Autodesk Fusion 360 part; units mm, degrees
sketch "スケッチ1" plane through (0, 0, 0) normal (0, 0, 1) x (1, 0, 0)
  line L0 (-16.5, 22) -> (16.5, 22)
  line L1 (16.5, 22) -> (16.5, 0)
  line L2 (16.5, 0) -> (-16.5, 0)
  line L3 (-16.5, 0) -> (-16.5, 22)
  dimension "d7" = 22
  dimension "d8" = 33
extrude "押し出し1" add sketch "スケッチ1" along normal blind 2
sketch "スケッチ3" plane through (0, 0, 0) normal (0, 0, -1) x (1, 0, 0)
  line L0 (16.5, 0) -> (-16.5, 0)
  line L1 (-16.5, 0) -> (-16.5, -22)
  line L2 (-16.5, -22) -> (16.5, -22)
  line L3 (16.5, -22) -> (16.5, 0)
  arc A0 (-4.95, -13) -> (4.95, -13) centre (0, -13) ccw
  line L4 (16.5, -13) -> (-16.5, -13)
  dimension "d9" = 9.9
  dimension "d10" = 9
extrude "押し出し2" add sketch "スケッチ3" along normal blind 2 contours L1 L2 L3 A0 L4
sketch "スケッチ4" plane through (0, 0, -2) normal (0, 0, -1) x (1, 0, 0)
  line L0 (-4.95, -13) -> (-16.5, -13)
  line L1 (-16.5, -13) -> (-16.5, -22)
  line L2 (-16.5, -22) -> (16.5, -22)
  line L3 (16.5, -22) -> (16.5, -13)
  line L4 (16.5, -13) -> (4.95, -13)
  arc A0 (-4.95, -13) -> (4.95, -13) centre (0, -13) ccw
  line L5 (16.5, -22) -> (0.6, -22)
  line L6 (0.6, -22) -> (0.6, -13)
  line L7 (0.6, -13) -> (16.5, -13)
  line L8 (16.5, -13) -> (16.5, -22)
  line L9 (-16.5, -22) -> (-0.6, -22)
  line L10 (-0.6, -22) -> (-0.6, -13)
  line L11 (-0.6, -13) -> (-16.5, -13)
  line L12 (-16.5, -13) -> (-16.5, -22)
  dimension "d13" = 1.2
extrude "押し出し3" add sketch "スケッチ4" along normal blind 2
sketch "スケッチ5" plane through (0, 0, 0) normal (0, 0, -1) x (1, 0, 0)
  line L0 (4.95, -13) -> (16.5, -13)
  line L1 (16.5, -13) -> (16.5, 0)
  line L2 (16.5, 0) -> (-16.5, 0)
  line L3 (-16.5, 0) -> (-16.5, -13)
  line L4 (-16.5, -13) -> (-4.95, -13)
  arc A0 (-4.95, -13) -> (4.95, -13) centre (0, -13) ccw
  line L5 (-3.75, 0) -> (3.75, 0)
  line L6 (3.75, 0) -> (3.75, -18)
  line L7 (3.75, -18) -> (-3.75, -18)
  line L8 (-3.75, -18) -> (-3.75, 0)
  line L9 (0, -1.75) -> (0, -22.5)
  line L10 (3.75, -7) -> (16.5, -7)
  line L11 (-3.75, -7) -> (-16.5, -7)
  dimension "d17" = 7.5
  dimension "d18" = 11
  dimension "d19" = 11
sketch "スケッチ9" plane through (0, 13, 0) normal (0, -1, 0) x (1, 0, 0)
  line L0 (-4.95, 0) -> (-16.5, 0)
  line L1 (-16.5, 0) -> (-16.5, -4)
  line L2 (-16.5, -4) -> (-0.6, -4)
  line L3 (-0.6, -4) -> (-0.6, -2)
  line L4 (-0.6, -2) -> (-4.95, -2)
  line L5 (-4.95, -2) -> (-4.95, 0)
  line L6 (-2, -2) -> (2, -2)
  line L7 (2, -2) -> (2, -4)
  line L8 (2, -4) -> (-2, -4)
  line L9 (-2, -4) -> (-2, -2)
  line L10 (16.5, -4) -> (0.6, -4)
  dimension "d37" = 4
  dimension "d38" = 2
extrude "押し出し7" cut sketch "スケッチ9" against normal blind 1.5 contours L2 L3 L4 L6 L8 L9 | L3 L6 L7 L8 L10
sketch "スケッチ11" plane through (0, 22, 0) normal (0, 1, 0) x (-1, 0, 0)
  line L0 (16.5, -4) -> (16.5, 2)
  line L1 (16.5, 2) -> (-16.5, 2)
  line L2 (-16.5, 2) -> (-16.5, -4)
  line L3 (-16.5, -4) -> (16.5, -4)
  line L4 (16.5, 2) -> (-13.5, 2)
  line L5 (-13.5, 2) -> (-13.5, 12)
  line L6 (-13.5, 12) -> (16.5, 12)
  line L7 (16.5, 12) -> (16.5, 2)
  dimension "d49" = 10
ref_plane "作業平面1" through (0, 11, -1) normal (0, 1, 0) x (-1, 0, 0)
sketch "スケッチ13" plane through (0, 11, -1) normal (0, 1, 0) x (1, 0, 0)
  line L0 (16.5, -10) -> (-16.5, -10)
  line L1 (-16.5, -10) -> (-16.5, -3)
  line L2 (-16.5, -3) -> (16.5, -3)
  line L3 (16.5, -3) -> (16.5, -10)
  line L4 (16.5, 3) -> (16.5, -3)
  line L5 (-16.5, 3) -> (-16.5, -3)
  circle A0 centre (0, -6.5) radius 2.25
  dimension "d53" = 7
  dimension "d54" = 4.5
  dimension "d58" = 3.5
extrude "押し出し11" add sketch "スケッチ13" along normal blind -2 and the other way blind -8
sketch "Sketch17" plane through (16.5, 0, 0) normal (1, 0, 0) x (0, 1, 0)
  line L0 (22, -4) -> (22, 2)
  line L1 (22, 2) -> (19, 2)
  line L2 (19, 2) -> (19, 9)
  line L3 (19, 9) -> (9, 9)
  line L4 (9, 9) -> (9, 2)
  line L5 (9, 2) -> (0, 2)
  line L6 (0, 2) -> (0, 0)
  line L7 (0, 0) -> (13, 0)
  line L8 (13, 0) -> (13, -4)
  line L9 (13, -4) -> (22, -4)
  line L10 (11, 9) -> (17, 9)
  line L11 (17, 9) -> (17, 2)
  line L12 (17, 2) -> (11, 2)
  line L13 (11, 2) -> (11, 9)
extrude "Extrude15" cut sketch "Sketch17" against normal blind 400 contours L3 L10 L11 L12 L13
sketch "Sketch18" plane through (-16.5, 0, 0) normal (-1, 0, 0) x (0, -1, 0)
  line L0 (-11, 9) -> (-11, 2)
  line L1 (-11, 2) -> (-17, 2)
  line L2 (-17, 2) -> (-17, 9)
  line L3 (-17, 9) -> (-19, 9)
  line L4 (-19, 9) -> (-19, 2)
  line L5 (-19, 2) -> (-22, 2)
  line L6 (-22, 2) -> (-22, -4)
  line L7 (-22, -4) -> (-13, -4)
  line L8 (-13, -4) -> (-13, 0)
  line L9 (-13, 0) -> (0, 0)
  line L10 (0, 0) -> (0, 2)
  line L11 (0, 2) -> (-9, 2)
  line L12 (-9, 2) -> (-9, 9)
  line L13 (-9, 9) -> (-11, 9)
  line L14 (-9, 2) -> (0, 2)
  line L15 (0, 2) -> (0, 0)
  line L16 (0, 0) -> (-9, 0)
  line L17 (-9, 0) -> (-9, 2)
extrude "Extrude16" cut sketch "Sketch18" against normal blind 34 contours L9 L10 L11 L14 L15 L16 L17
sketch "Sketch19" plane through (0, 13, 0) normal (0, -1, 0) x (1, 0, 0)
  line L0 (2, -2) -> (2, -4)
  line L1 (2, -4) -> (16.5, -4)
  line L2 (16.5, -4) -> (16.5, 0)
  line L3 (16.5, 0) -> (4.95, 0)
  line L4 (4.95, 0) -> (4.95, -2)
  line L5 (4.95, -2) -> (2, -2)
  line L6 (0.6, -2) -> (16.5, -2)
  line L7 (-0.6, -2) -> (-16.5, -2)
  point P0 (12, -2)
  point P1 (-12, -2)
hole "Hole1" at (-12, 13, -2) at (12, 13, -2) direction (0, 1, 0) diameter 2.75 depth 5 tip angle 118
sketch "Sketch20" plane through (0, 9, 0) normal (0, -1, 0) x (1, 0, 0)
  circle A0 centre (0, 5.5) radius 2.25
  line L0 (16.5, 0) -> (16.5, 9)
  line L1 (16.5, 9) -> (-16.5, 9)
  line L2 (-16.5, 9) -> (-16.5, 0)
  line L3 (-16.5, 0) -> (16.5, 0)
  circle A1 centre (0, 5) radius 4
  curve L4
  curve L5
  curve L6
  curve L7
  line L8 (-16.5, 2.0263) -> (16.5, 2.0263)
  line L9 (16.5, 2.0263) -> (16.5, 0)
  line L10 (16.5, 0) -> (-16.5, 0)
  line L11 (-16.5, 0) -> (-16.5, 2.0263)
  line L12 (-4, 5) -> (-4, 2.0263)
  line L13 (4, 5) -> (4, 2.0263)
  point P0 (-16.5, 2)
extrude "Extrude17" cut sketch "Sketch20" against normal blind 150 contours L0 L1 A1 L8 L13 | L1 L2 A1 L8 L12
sketch "Sketch21" plane through (0, 0, -4) normal (0, 0, -1) x (1, 0, 0)
  line L0 (2, -13) -> (2, -14.5)
  line L1 (2, -14.5) -> (0.6, -14.5)
  line L2 (0.6, -14.5) -> (0.6, -17.9135)
  arc A0 (-0.6, -17.9135) -> (0.6, -17.9135) centre (0, -13) ccw
  line L3 (-0.6, -17.9135) -> (-0.6, -14.5)
  line L4 (-0.6, -14.5) -> (-2, -14.5)
  line L5 (-2, -14.5) -> (-2, -13)
  line L6 (-2, -13) -> (-16.5, -13)
  line L7 (-16.5, -13) -> (-16.5, -22)
  line L8 (-16.5, -22) -> (16.5, -22)
  line L9 (16.5, -22) -> (16.5, -13)
  line L10 (16.5, -13) -> (2, -13)
sketch "Sketch22" plane through (0, 0, 0) normal (0, 0, -1) x (1, 0, 0)
  line L0 (16.5, -9) -> (-16.5, -9)
  line L1 (-16.5, -9) -> (-16.5, -13)
  line L2 (-16.5, -13) -> (-4.95, -13)
  arc A0 (-4.95, -13) -> (4.95, -13) centre (0, -13) ccw
  line L3 (4.95, -13) -> (16.5, -13)
  line L4 (16.5, -13) -> (16.5, -9)
  circle A1 centre (0, -13) radius 9
extrude "Extrude18" cut sketch "Sketch22" against normal blind 10 contours L0 L3 L4 A1 | L0 L1 L2 A1
move_face "OffsetFaces1" offset -1 1 faces at (16.5, 17.3333, -2)
move_face "OffsetFaces2" offset -0.5 1 faces at (15.5, 17.3333, -2)
move_face "OffsetFaces3" offset -1.5 1 faces at (-16.5, 17.3333, -2)
move_face "OffsetFaces4" offset 1 1 faces at (5, 22, 0)
move_face "OffsetFaces5" offset -1 1 faces at (5, 23, 0)
Here's how the part is built. I have some questions about the finished solid (model axes, mm). A direction names the side the tool comes from. Coordinates: 2 decimals unless noted, no trailing zeros. Order: outer loops, then holes, each group sorted by start corner. A loop starts at its lowest first (then second) coordinate and runs counter-clockwise, first axis right, second up. Notation, with made-up numbers: (76, 61) -> (127, 61) arc R12 ccw to (127, 84) -> close; hole circle Ø8 at (72.5, 79.5). An arc over 180 degrees is marked (long way). Return JSON: item names as keys, results as strings.
1) If we section it at C-C on z = 1.25: List the corners of the cut face in (x, y) for me.
Conclusion:
{"outline": "(-15, 13) -> (-9, 13) arc R9 ccw to (-8.06, 9) -> (8.06, 9) arc R9 ccw to (9, 13) -> (15, 13) -> (15, 22) -> (-15, 22) -> close"}
2) I'm going to push flat-ended pins straight in: P1, Ø0.6, axis at x = 5.5, y = 9.5, coming from the +Z side; P2, Ø3, axis at y = 20, z = 4, coming from the -X side; P3, Ø7.5, axis at x = 1, z = 6.5, coming from the +Y side. Where does each tip first touch, or does it pass through?
Conclusion:
{"P1": "stops at z = 2.03", "P2": "stops at x = -4", "P3": "stops at y = 19"}
3) Thinking about a two-plate mould opening in Y: for faces 1 (the flat face through (0, 15, 2)), 2 (the flat face through (4, 10, 4)), 3 (the flat face through (1, 14.5, -3)), which applies, +Y half, -Y half, draft (parallel to the pull), parting line (faces both ways), or undercut?
Conclusion:
{"face 1": "undercut", "face 2": "draft", "face 3": "-Y half"}
4) If I drill on probe 1 along Y at (x, z) = (3, 5); probe 2 along Z at (x, y) = (-3.25, 15.25); probe 3 along Z at (x, y) = (12, 14.7) (3 decimals), over which ranges is the centre line in solid material (lowest first)?
Conclusion:
{"probe 1": "y = 9 to 11, 17 to 19", "probe 2": "z = -4 to -2, 0 to 2", "probe 3": "z = -4 to -3.375, -0.625 to 2"}
5) On a 3-axis mill with a long thin cutter (end or side, diameter ignored), from which of +Z, -Z, +X, -X, +Y, -Y can I reach the whole of each face in a straight line? I mean faces 4 (the flat face through (-2, 14, -3)), 5 (the flat face through (0, 21, 2)), 6 (the flat face through (-3, 15, -2)), 7 (the flat face through (4, 18, 4)). Say none if no direction works.
Conclusion:
{"face 4": "-Z, -Y", "face 5": "+Z, +X, -X, +Y", "face 6": "-Y", "face 7": "+Z, +X, +Y, -Y"}
6) If we section it at A-A on x = 0: List the corners of the cut face in (y, z) for me.
Conclusion:
{"outline": "(9, 0) -> (17.95, 0) -> (17.95, -4) -> (22, -4) -> (22, 2) -> (19, 2) -> (19, 3.25) -> (17, 3.25) -> (17, 2) -> (11, 2) -> (11, 3.25) -> (9, 3.25) -> close; (9, 7.75) -> (11, 7.75) -> (11, 9) -> (9, 9) -> close; (17, 7.75) -> (19, 7.75) -> (19, 9) -> (17, 9) -> close"}
7) If we section it at B-B on z = 4.5: List the corners of the cut face in (x, y) for me, plus the area to 3 significant figures.
Conclusion:
{"outline": "(-4, 9) -> (-2.02, 9) -> (-2.02, 11) -> (-4, 11) -> close; (-4, 17) -> (-2.02, 17) -> (-2.02, 19) -> (-4, 19) -> close; (2.02, 9) -> (4, 9) -> (4, 11) -> (2.02, 11) -> close; (2.02, 17) -> (4, 17) -> (4, 19) -> (2.02, 19) -> close", "area": "15.9 mm²"}
8) If we section it at D-D on x = -3.5: List the corners of the cut face in (y, z) for me, plus the area to 3 significant figures.
Conclusion:
{"outline": "(9, 0) -> (16.5, 0) -> (16.5, -2) -> (13, -2) -> (13, -4) -> (22, -4) -> (22, 2) -> (19, 2) -> (19, 6.94) -> (17, 6.94) -> (17, 2) -> (11, 2) -> (11, 6.94) -> (9, 6.94) -> close", "area": "74.7 mm²"}
